```python
from build123d import *

# Parameters (mm, degrees)
BOSS_EXTRUDE1_DEPTH      = 12
BOSS_EXTRUDE2_DEPTH      = 6
BOSS_EXTRUDE2_DEPTH_BACK = 6
SKETCH3_R                = 14.5
BOSS_EXTRUDE3_DEPTH      = 19.9
BOSS_EXTRUDE3_DEPTH_BACK = 19.9
SKETCH4_W                = 134
SKETCH4_H                = 102
CUT_EXTRUDE1_DEPTH       = 1.2


with BuildPart() as part:
    # Sketch1 → Boss-Extrude1 (new body)
    with BuildSketch(Plane(origin=(0, 0, 0), x_dir=(1, 0, 0), z_dir=(0, 1, 0))):
        with BuildLine():
            Line((-25.5, -25.5), (25.5, -25.5))
            ThreePointArc((25.5, -25.5), (31.156854249, -23.156854249), (33.5, -17.5))
            Line((33.5, -17.5), (33.5, 17.5))
            ThreePointArc((33.5, 17.5), (31.156854249, 23.156854249), (25.5, 25.5))
            Line((25.5, 25.5), (-25.5, 25.5))
            ThreePointArc((-25.5, 25.5), (-31.156854249, 23.156854249), (-33.5, 17.5))
            Line((-33.5, 17.5), (-33.5, -17.5))
            ThreePointArc((-33.5, -17.5), (-31.156854249, -23.156854249), (-25.5, -25.5))
        make_face()
    extrude(amount=BOSS_EXTRUDE1_DEPTH)

    # Sketch2 → Boss-Extrude2 (add, two sides)
    with BuildSketch(Plane(origin=(0, 0, 0), x_dir=(0, 0, -1), z_dir=(1, 0, 0))) as boss_extrude2_sk:
        Polygon((-33.505924481, 46.247123846), (-24.329435304, 12), (19.182468036, 12), (-6.942631645, 57.25), align=None)
    extrude(amount=BOSS_EXTRUDE2_DEPTH)
    extrude(boss_extrude2_sk.sketch, amount=-BOSS_EXTRUDE2_DEPTH_BACK)

    # Sketch3 → Boss-Extrude3 (add, two sides)
    with BuildSketch(Plane(origin=(0, 0, 0), x_dir=(0, 0, -1), z_dir=(1, 0, 0))) as boss_extrude3_sk:
        with Locations((-19.5, 50)):
            Circle(SKETCH3_R)
    extrude(amount=BOSS_EXTRUDE3_DEPTH)
    extrude(boss_extrude3_sk.sketch, amount=-BOSS_EXTRUDE3_DEPTH_BACK)

    # Sketch4 → Cut-Extrude1 (cut)
    with BuildSketch(Plane(origin=(0, 12, 0), x_dir=(1, 0, 0), z_dir=(0, 1, 0))):
        Rectangle(SKETCH4_W, SKETCH4_H)
        with BuildLine():
            Line((-33.5, 16.5), (-33.5, -16.5))
            Line((-33.5, -16.5), (-33.237991266, -15.534934498))
            ThreePointArc((-33.237991266, -15.534934498), (-21.607110594, -11.421141335), (-21.862465515, -23.755462284))
            Line((-21.862465515, -23.755462284), (-24.5, -25.5))
            Line((-24.5, -25.5), (24.5, -25.5))
            Line((24.5, -25.5), (21.862465515, -23.755462284))
            ThreePointArc((21.862465515, -23.755462284), (21.607110594, -11.421141335), (33.237991266, -15.534934498))
            Line((33.237991266, -15.534934498), (33.5, -16.5))
            Line((33.5, -16.5), (33.5, 16.5))
            Line((33.5, 16.5), (33.237991266, 15.534934498))
            ThreePointArc((33.237991266, 15.534934498), (21.607110594, 11.421141335), (21.862465515, 23.755462284))
            Line((21.862465515, 23.755462284), (24.5, 25.5))
            Line((24.5, 25.5), (-24.5, 25.5))
            Line((-24.5, 25.5), (-21.862465515, 23.755462284))
            ThreePointArc((-21.862465515, 23.755462284), (-21.607110594, 11.421141335), (-33.237991266, 15.534934498))
            Line((-33.237991266, 15.534934498), (-33.5, 16.5))
        make_face(mode=Mode.SUBTRACT)
    extrude(amount=-CUT_EXTRUDE1_DEPTH, mode=Mode.SUBTRACT)

    # Sketch5 → Cut-Revolve1 (revolve, cut)
    with BuildSketch(Plane.XY.offset(17.5)):
        Polygon((-26, 0), (-30.5, 0), (-30.5, 10.8), (-33.5, 10.8), (-33.5, 12), (-26, 12), align=None)
    revolve(axis=Axis((-26, 12, 17.5), (0, -1, 0)), mode=Mode.SUBTRACT)

    # Sketch6 → Cut-Revolve2 (revolve, cut)
    with BuildSketch(Plane.XY.offset(-17.5)):
        Polygon((-26, 0), (-30.5, 0), (-30.5, 10.8), (-33.5, 10.8), (-33.5, 12), (-26, 12), align=None)
    revolve(axis=Axis((-26, 12, -17.5), (0, -1, 0)), mode=Mode.SUBTRACT)

    # Sketch7 → Cut-Revolve3 (revolve, cut)
    with BuildSketch(Plane.XY.offset(17.5)):
        Polygon((26, 0), (21.5, 0), (21.5, 10.8), (18.5, 10.8), (18.5, 12), (26, 12), align=None)
    revolve(axis=Axis((26, 12, 17.5), (0, -1, 0)), mode=Mode.SUBTRACT)

    # Sketch8 → Cut-Revolve4 (revolve, cut)
    with BuildSketch(Plane.XY.offset(-17.5)):
        Polygon((26, 0), (21.5, 0), (21.5, 10.8), (18.5, 10.8), (18.5, 12), (26, 12), align=None)
    revolve(axis=Axis((26, 12, -17.5), (0, -1, 0)), mode=Mode.SUBTRACT)

    # Sketch9 → Cut-Revolve5 (revolve, cut)
    with BuildSketch(Plane.XY.offset(19.5)):
        Polygon((-19.9, 50), (-19.9, 61.5), (-19.611324865, 61), (19.611324865, 61), (19.9, 61.5), (19.9, 50), align=None)
    revolve(axis=Axis((19.9, 50, 19.5), (-1, 0, 0)), mode=Mode.SUBTRACT)

    # Sketch10 → Revolve1 (revolve)
    with BuildSketch(Plane.XY.offset(19.5)):
        Polygon((-19.9, 58.3), (-19.6, 58), (19.6, 58), (19.9, 58.3), (19.9, 60.7), (19.6, 61), (-19.6, 61), (-19.9, 60.7), align=None)
    revolve(axis=Axis((19.9, 50, 19.5), (-1, 0, 0)))


solid = part.part
```
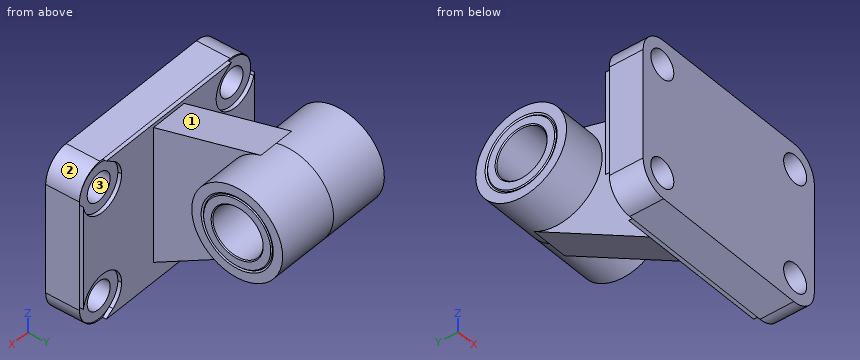
For this review, take the finished solid that the model builds, in its own axes (mm). Face numbers are marked on the shaded views. Coordinates: 2 decimals unless noted, no trailing zeros. Loops run counter-clockwise (first coordinate to the right, second up) from the corner with the lowest first, then second, coordinate; pieces in that order, holes last.
1. Mouldability with a two-part tool opening along X and no side actions: class the marked faces 1, 2 and 3 as +X half, -X half, draft (parallel to the pull), parting line (faces both ways), or undercut.
2. Insertion check: P1, Ø4, axis at y = 29.5, z = 20, coming from the +X side; P2, Ø17, axis at y = 47.5, z = 15.5, coming from the +X side; P3, Ø16.5, axis at x = -28.5, z = -15.5, coming from the +Y side. Each pin has a flat end and moves straight along its axis. Give the tip position at first contact, or say it passes through.
3. Add section C-C, the plane z = -6. Give the boundary of the cut face in (x, y), then the cut area to 3 significant figures.
4. Add section D-D, the plane y = 19. Give the boundary of the cut face in (x, z), then the cut area to 3 significant figures.
5. Add section A-A, the plane x = 15. Give the boundary of the cut face in (y, z), then the cut area to 3 significant figures.
6. For line 1 (Y direction, x = -19.55, z = 19.5); line 2 (Z direction, x = -26, y = 3); line 3 (Z direction, x = -19, y = 50), list the stretches that pass through material, from the lowest coordinate up.
Result:
1. face 1: draft
1. face 2: +X half
1. face 3: undercut
2. P1: stops at x = 6
2. P2: stops at x = 19.9
2. P3: stops at y = 12
3. outline: (-33.5, 0) - (33.5, 0) - (33.5, 12) - (6, 12) - (6, 34.83) - (-6, 34.83) - (-6, 12) - (-33.5, 12) - close
3. area: 1,080 mm2
4. outline: (-6, -15.14) - (6, -15.14) - (6, 26.21) - (-6, 26.21) - close
4. area: 496 mm2
5. outline: (0, -25.5) - (12, -25.5) - (12, 25.5) - (0, 25.5) - close; circle Ø29 at (50, 19.5); hole circle Ø16 at (50, 19.5)
5. area: 1,070 mm2
6. line 1: y = 0 to 10.8, 35.5 to 42, 58 to 64.5
6. line 2: z = -25.48 to -22, -13 to 13, 22 to 25.48
6. line 3: z = 5 to 11.5, 27.5 to 34
